```python
from build123d import *

# Parameters (mm, degrees)
SKETCH1_W             = 8.89
SKETCH1_H             = 8.89
BASE_FLANGE1_DEPTH    = 0.9144
F_2_CLEARANCE_HOLE1_D = 2.4384


# Sheet-metal steps are written as plain solids
with BuildPart() as part:
    # Sketch1 → Base-Flange1 (new body)
    with BuildSketch(Plane(origin=(0, 0, 0), x_dir=(1, 0, 0), z_dir=(0, 1, 0))):
        with Locations((4.445, 4.445)):
            Rectangle(SKETCH1_W, SKETCH1_H)
    extrude(amount=-BASE_FLANGE1_DEPTH)

    # #2 Clearance Hole1 (through all)
    with Locations(Plane(origin=(0, 0, 0), x_dir=(1, 0, 0), z_dir=(0, 1, 0))):
        with Locations((6.858, 2.54), (6.858, 6.35)):
            Hole(F_2_CLEARANCE_HOLE1_D / 2)


solid = part.part
```
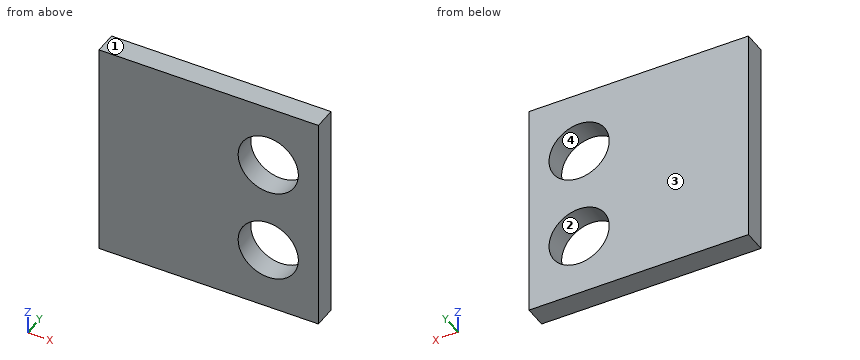
Verification items for the finished model (mm, model axes). Face numbers are marked on the shaded views. Give positions to 0.01 mm unless a question says otherwise; leave off trailing zeros. Order: outer loops, then holes, each group sorted by start corner. A loop starts at its lowest first (then second) coordinate and runs counter-clockwise, first axis right, second up. Notation, with made-up numbers: M 47.5,64.5 L 85.5,64.5 A16 ccw 85.5,90.5 Z; hole C -31.75,86 d4. An arc over 180 degrees is marked long. Return JSON: item names as keys, results as strings. Group by question number.
1) Section check B-B on x = 5.75. Record the cut outline in (y, z).
2) Section check C-C on y = -0.7. Record the cut outline in (x, z), and give its area (3 significant figures).
3) Scan lines: line 1 (X direction, y = -0.55, z = -6.35); line 2 (Z direction, x = 5.75, y = -0.15); line 3 (Z direction, x = 7, y = -0.8). Record each from-to range of solid material in increasing order.
4) Go/stop test with a flat-tipped pin: pin 1 Ø5 at (x, z) = (7.5, -7) entering from +Y. Record where the tip stops, or that it passes through.
5) Section check D-D on x = 7. Record the cut outline in (y, z).
6) Mould release check, pull along Z, two halves, no side actions. Record for the marked faces 1, 2, 3 and 4: pulls with the +Z half, pulls with the -Z half, needs draft (parallel to the pull), parting line crosses it, or undercut.
7) Section check A-A on z = -2.54. Record the cut outline in (x, y).
Answer block:
{
 "1": {"outline": "M -0.91,-8.89 L 0,-8.89 L 0,-6.86 L -0.91,-6.86 Z; M -0.91,-5.84 L 0,-5.84 L 0,-3.05 L -0.91,-3.05 Z; M -0.91,-2.03 L 0,-2.03 L 0,0 L -0.91,0 Z"},
 "2": {"outline": "M 0,-8.89 L 8.89,-8.89 L 8.89,0 L 0,0 Z; hole C 6.86,-6.35 d2.44; hole C 6.86,-2.54 d2.44", "area": "69.7 mm^2"},
 "3": {"line 1": "x = 0 to 5.64, 8.08 to 8.89", "line 2": "z = -8.89 to -6.86, -5.84 to -3.05, -2.03 to 0", "line 3": "z = -8.89 to -7.56, -5.14 to -3.75, -1.33 to 0"},
 "4": {"pin 1": "stops at y = 0"},
 "5": {"outline": "M -0.91,-8.89 L 0,-8.89 L 0,-7.56 L -0.91,-7.56 Z; M -0.91,-5.14 L 0,-5.14 L 0,-3.75 L -0.91,-3.75 Z; M -0.91,-1.33 L 0,-1.33 L 0,0 L -0.91,0 Z"},
 "6": {"face 1": "pulls with the +Z half", "face 2": "undercut", "face 3": "needs draft", "face 4": "undercut"},
 "7": {"outline": "M 0,-0.91 L 5.64,-0.91 L 5.64,0 L 0,0 Z; M 8.08,-0.91 L 8.89,-0.91 L 8.89,0 L 8.08,0 Z"}
}
